Could you check a few things on this model? Use its own coordinates, in mm. A direction names the side the tool comes from. Coordinates: 2 decimals unless noted, no trailing zeros. Write each loop counter-clockwise with the first axis right and the second up, starting at its lowest first coordinate (ties: lowest second). Pieces come first, ordered by that corner, then holes. Notation, with made-up numbers: (85, -11) - (116, -11) arc R25 cw to (116, 20) - close; hole circle Ø5 at (-29.75, 61). An arc over 180 degrees is marked (long way). Answer as a JSON object with one key per item and string values. Group by question number.
1) If we section it at B-B (y = 0): Write out the boundary of the cut face in (x, z) (1 decimal).
2) If we section it at C-C (z = 6.35): Write out the boundary of the cut face in (x, y).
3) Will these pins go through, and if not, where does the flat tip stop? pin 1 Ø4 at (y, z) = (5.5, 2) entering from +X; pin 2 Ø0.5 at (x, z) = (18.5, 9) entering from -Y; pin 3 Ø0.6 at (x, y) = (13.5, 16.5) entering from +Z (3 decimals).
4) If we section it at A-A (x = 0): Write out the boundary of the cut face in (y, z), plus the area to 3 significant figures.
5) Please list where these lines run through material, in increasing order: line 1 along Y through (x, z) = (0, 2.75); line 2 along X through (y, z) = (-0.5, 2.25); line 3 along X through (y, z) = (11, 8.75).
6) On a 3-axis mill with a long thin cutter (end or side, diameter ignored), from which of +Z, -Z, +X, -X, +Y, -Y can I reach the whole of each face in a straight line? I mean faces 4 (the flat face through (13, 17.62, 9)), 5 (the flat face through (20.822, -16, 9)), 6 (the flat face through (15, -10.537, 9)), 7 (the flat face through (9.18, -16.307, 10.196)). Say none if no direction works.
7) We'd pull the mould along X, two halves only. Please class faces 1 (the flat face through (17, 0, 7.62)), 2 (the flat face through (50.8, 0, 6)), 3 (the flat face through (-37, 0, 12.7)): released by +X, released by -X, zero draft, split by the parting line, or undercut.
```python
from build123d import *

# Parameters (mm, degrees)
F0_W      = 76.2
F0_H      = 50.8
F0_R      = 12.7
F1_DEPTH  = 12.7
F2_W      = 6.35
F2_H      = 50.8
F3_DEPTH  = 2.54
F5_DEPTH  = 50.801
F6_R      = 4.7625
F7_DEPTH  = 12.7
F8_W      = 2.186066
F8_H      = 2.098622
F8_W_2    = 2.360951
F8_H_2    = 2.798164
F8_W_3    = 2.448395
F8_H_3    = 2.273508
F8_H_4    = 2.186067
F9_DEPTH  = 1.905
F10_W     = 0.841629
F10_H     = 0.611811
F10_W_2   = 0.649078
F10_H_2   = 0.581
F11_DEPTH = 0.0762
F12_W     = 0.539394
F12_H     = 0.506463
F12_W_2   = 0.672908
F12_H_2   = 0.530849
F13_DEPTH = 0.0762
F14_W     = 0.521662
F14_H     = 0.444038
F14_W_2   = 0.538152
F14_H_2   = 0.436696
F15_DEPTH = 0.0762
F16_W     = 0.567031
F16_H     = 0.357919
F16_W_2   = 0.504408
F16_H_2   = 0.379607
F17_DEPTH = 0.0762


with BuildPart() as f1:
    # F0 (on Top) → F1 (new body)
    with BuildSketch(Plane.XY):
        Rectangle(F0_W, F0_H)
        Circle(F0_R, mode=Mode.SUBTRACT)
    extrude(amount=F1_DEPTH)

    # F2 (on face) → F3 (cut)
    with BuildSketch(Plane.XY.offset(12.7)):
        with Locations((-32.385, 0)):
            Rectangle(F2_W, F2_H)
        with BuildLine():
            Line((-4.147136, -12.003802), (-4.147136, -25.4))
            Line((-4.147136, -25.4), (8.552864, -25.4))
            Line((8.552864, -25.4), (8.552864, -9.388212))
            ThreePointArc((8.552864, -9.388212), (2.561823, -12.438933), (-4.147136, -12.003802))
        make_face()
        with BuildLine():
            Line((8.552864, 25.4), (-4.147136, 25.4))
            Line((-4.147136, 25.4), (-4.147136, 12.003802))
            ThreePointArc((-4.147136, 12.003802), (2.561823, 12.438933), (8.552864, 9.388212))
            Line((8.552864, 9.388212), (8.552864, 25.4))
        make_face()
    extrude(amount=-F3_DEPTH, mode=Mode.SUBTRACT)

    # F4 (on face) → F5 (cut, through all)
    with BuildSketch(Plane.XZ.offset(25.4)):
        Polygon((23.326432, 12.7), (10.626432, 12.7), (7.693492, 7.62), (26.259371, 7.62), align=None)
    extrude(amount=-F5_DEPTH, mode=Mode.SUBTRACT)

    # F6 (on face) → F7 (join)
    with BuildSketch(Plane.YZ.offset(38.1)):
        with Locations((0, 6.35)):
            Circle(F6_R)
    extrude(amount=F7_DEPTH)

    # F8 (on face) → F9 (join)
    with BuildSketch(Plane.XY.offset(7.62)):
        with Locations((13.345409, 16.570377)):
            Rectangle(F8_W, F8_H)
        with Locations((19.204065, 0.393492)):
            Rectangle(F8_W_2, F8_H_2)
        with Locations((14.788213, -11.67359)):
            Rectangle(F8_W_3, F8_H_3)
        with Locations((19.597556, -16.176885)):
            Rectangle(F8_W_3, F8_H_4)
    extrude(amount=F9_DEPTH)

    # F10 (on face) → F11 (cut)
    with BuildSketch(Plane.XZ.offset(17.269919)):
        with Locations((20.068542, 8.770566)):
            Rectangle(F10_W, F10_H)
        with Locations((18.937801, 8.785971)):
            Rectangle(F10_W_2, F10_H_2)
    extrude(amount=-F11_DEPTH, mode=Mode.SUBTRACT)

    # F12 (on face) → F13 (cut)
    with BuildSketch(Plane.XZ.offset(12.810344)):
        with Locations((14.095002, 8.64309)):
            Rectangle(F12_W, F12_H)
        with Locations((15.033044, 8.630897)):
            Rectangle(F12_W_2, F12_H_2)
    extrude(amount=-F13_DEPTH, mode=Mode.SUBTRACT)

    # F14 (on face) → F15 (cut)
    with BuildSketch(Plane.XZ.offset(1.00559)):
        with Locations((18.586445, 8.935527)):
            Rectangle(F14_W, F14_H)
        with Locations((19.417457, 8.939198)):
            Rectangle(F14_W_2, F14_H_2)
    extrude(amount=-F15_DEPTH, mode=Mode.SUBTRACT)

    # F16 (on face) → F17 (cut)
    with BuildSketch(Plane.XZ.offset(-15.521066)):
        with Locations((12.797092, 8.772087)):
            Rectangle(F16_W, F16_H)
        with Locations((13.668423, 8.761243)):
            Rectangle(F16_W_2, F16_H_2)
    extrude(amount=-F17_DEPTH, mode=Mode.SUBTRACT)


solid = f1.part
```
Here are the results:
{
 "1": {"outline": "(-38.1, 0) - (-12.7, 0) - (-12.7, 12.7) - (-29.2, 12.7) - (-29.2, 10.2) - (-35.6, 10.2) - (-35.6, 12.7) - (-38.1, 12.7) - close; (12.7, 0) - (38.1, 0) - (38.1, 1.6) - (50.8, 1.6) - (50.8, 11.1) - (38.1, 11.1) - (38.1, 12.7) - (23.3, 12.7) - (26.3, 7.6) - (20.4, 7.6) - (20.4, 9.5) - (18, 9.5) - (18, 7.6) - (12.7, 7.6) - close"},
 "2": {"outline": "(-38.1, -25.4) - (38.1, -25.4) - (38.1, -4.76) - (50.8, -4.76) - (50.8, 4.76) - (38.1, 4.76) - (38.1, 25.4) - (-38.1, 25.4) - close; hole circle Ø25.4 at (0, 0)"},
 "3": {"pin 1": "stops at x = 38.1", "pin 2": "stops at y = -17.27", "pin 3": "stops at z = 9.525"},
 "4": {"outline": "(-25.4, 0) - (-12.7, 0) - (-12.7, 10.16) - (-25.4, 10.16) - close; (12.7, 0) - (25.4, 0) - (25.4, 10.16) - (12.7, 10.16) - close", "area": "258 mm²"},
 "5": {"line 1": "y = -25.4 to -12.7, 12.7 to 25.4", "line 2": "x = -38.1 to -12.69, 12.69 to 50.8", "line 3": "x = -38.1 to -6.35, 6.35 to 8.35, 25.61 to 38.1"},
 "6": {"face 4": "+Z, +Y", "face 5": "+Z, +Y, -Y", "face 6": "+Z", "face 7": "+Y, -Y"},
 "7": {"face 1": "undercut", "face 2": "released by +X", "face 3": "zero draft"}
}
